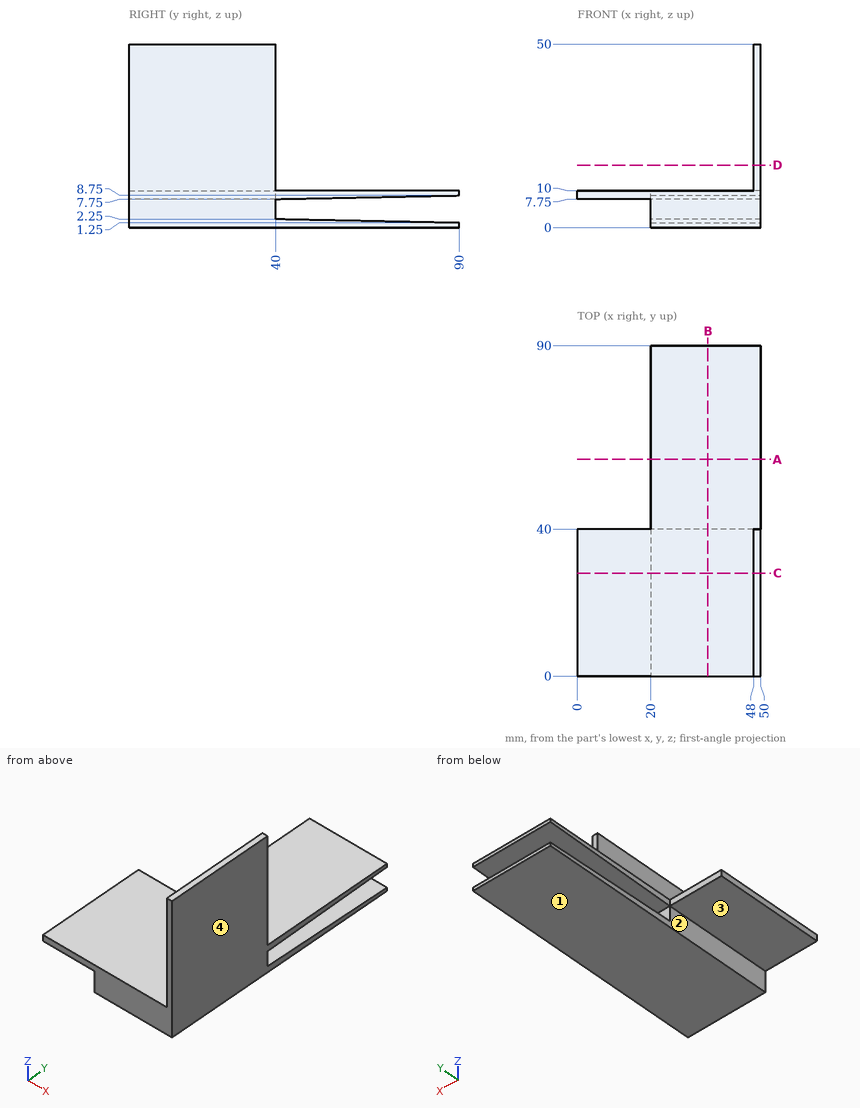
Here's the drawing with two shaded views (mm, measured from the low corner). I have some questions. A direction names the side the tool comes from. Round coordinates to 2 decimals unless told otherwise and drop trailing zeros. Loops run counter-clockwise (first coordinate to the right, second up) from the corner with the lowest first, then second, coordinate; pieces in that order, holes last. Notation, with made-up numbers: (42, 59.5) - (92, 59.5) arc R18 ccw to (92, 85.5) - close; hole circle Ø3 at (89.25, 38.25). An arc over 180 degrees is marked (long way). Write item = value, one per line.
1) On a 3-axis mill with a long thin cutter (end or side, diameter ignored), from which of +Z, -Z, +X, -X, +Y, -Y can I reach the whole of each face in a straight line? I mean the marked faces 1 and 2. Say none if no direction works.
Computed:
face_1 = -Z, +X, -X, +Y, -Y
face_2 = -Z, -X, +Y, -Y
2) Imagine slicing it at A-A (y = 59). Please give me the cut outline in (x, z), and give its area (3 significant figures).
Computed:
outline = (20, 0) - (50, 0) - (50, 1.87) - (20, 1.87) - close; (20, 8.13) - (50, 8.13) - (50, 10) - (20, 10) - close
area = 112 mm2
3) If we mould it in two halves opening along Z, with no side actions, what happens to the marked faces 3 and 4? For each: pulls with the +Z half, pulls with the -Z half, needs draft (parallel to the pull), parting line crosses it, or undercut.
Computed:
face_3 = pulls with the -Z half
face_4 = needs draft
4) Imagine slicing it at C-C (y = 28). Please give me the cut outline in (x, z).
Computed:
outline = (0, 7.75) - (20, 7.75) - (20, 0) - (50, 0) - (50, 50) - (48, 50) - (48, 10) - (0, 10) - close
5) Imagine slicing it at B-B (x = 35.5). Please give me the cut outline in (y, z).
Computed:
outline = (0, 0) - (90, 0) - (90, 1.25) - (40, 2.25) - (40, 7.75) - (90, 8.75) - (90, 10) - (0, 10) - close
6) I need wall thicknesses on line 1 along Z through (x, y) = (26.5, 8); line 2 along Z through (x, y) = (4, 20); line 3 along X through (y, z) = (26, 16). Which ranges of each line are inside material? Lowest first, please. Write a range as from..to.
Computed:
line_1 = 0..10
line_2 = 7.75..10
line_3 = 48..50
7) I'm going to push flat-ended pins straight in: P1, Ø0.6, axis at x = 49, z = 35, coming from the +Y side; P2, Ø8.5, axis at y = 54, z = 2, coming from the -X side; P3, Ø6, axis at x = 12.5, y = 22, coming from the -Z side. Where does each tip first touch, or does it pass through?
Computed:
P1 = 40
P2 = 20
P3 = 7.75
8) Imagine slicing it at D-D (z = 17). Please give me the cut outline in (x, y).
Computed:
outline = (48, 0) - (50, 0) - (50, 40) - (48, 40) - close
